Verification items for this drawing (mm, ordinates from the low corner). A direction names the side the tool comes from. Give positions to 0.01 mm unless a question says otherwise; leave off trailing zeros. Loops run counter-clockwise (first coordinate to the right, second up) from the corner with the lowest first, then second, coordinate; pieces in that order, holes last. Notation, with made-up numbers: (-33, -22.75) -> (10, -22.75) arc R18 cw to (10, 10.25) -> close; hole circle Ø7 at (26.25, -30). An arc over 180 degrees is marked (long way). Answer as a JSON object with one key per item and string values.
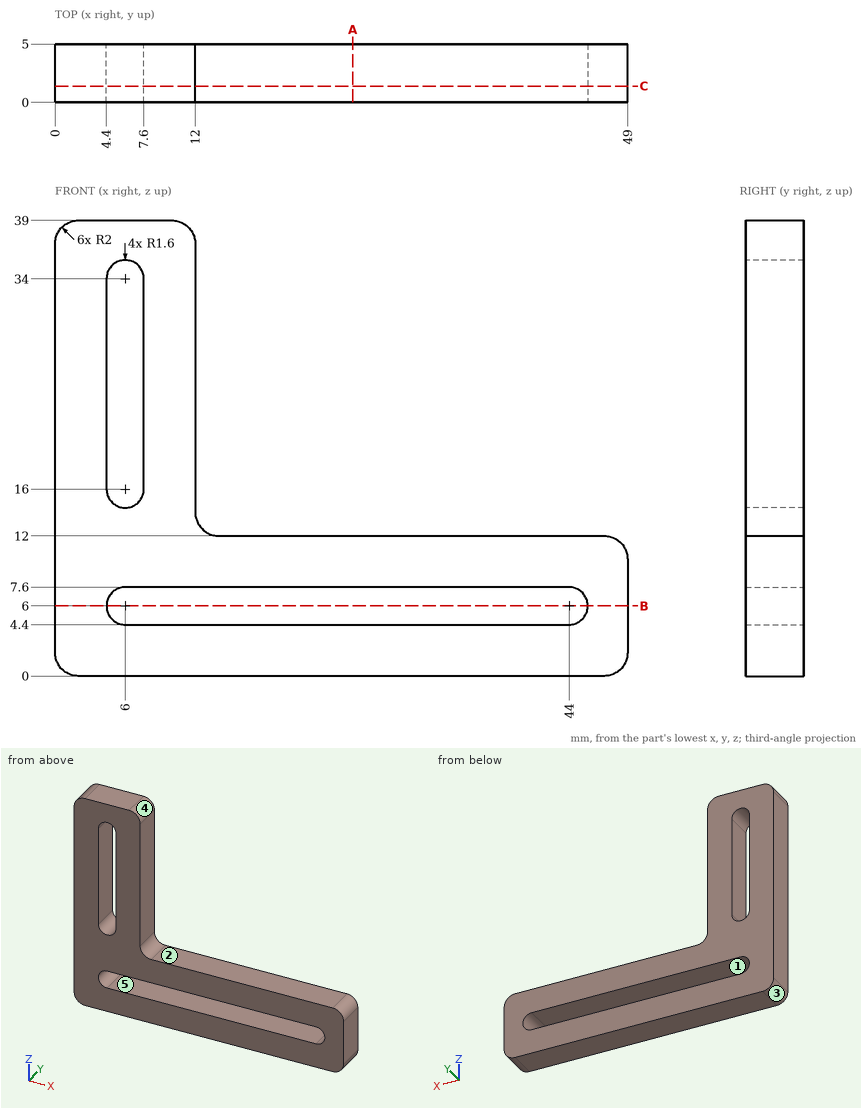
1) Tool access check on the marked faces 4 and 5. Record the directions out of +Z, -Z, +X, -X, +Y, -Y that give a thin tool (end or side, any length) a straight path to the whole face; none if there is none.
Geometry check:
{"face 4": "+Z, +X, +Y, -Y", "face 5": "+Y, -Y"}
2) Draft check along X on the marked faces 1, 2 and 3. Enter one of: pulls with the +X half, pulls with the -X half, needs draft (parallel to the pull), parting line crosses it, or undercut.
Geometry check:
{"face 1": "undercut", "face 2": "needs draft", "face 3": "pulls with the -X half"}
3) Section check A-A on x = 25.5. Record the cut outline in (y, z), plus the area to 3 significant figures.
Geometry check:
{"outline": "(0, 0) -> (5, 0) -> (5, 4.4) -> (0, 4.4) -> close; (0, 7.6) -> (5, 7.6) -> (5, 12) -> (0, 12) -> close", "area": "44.0 mm2"}
4) Material ranges on line 1 along X through (y, z) = (3.4, 24.5); line 2 along Z through (x, y) = (9, 2.5), recorded low to high. Write a range as from..to.
Geometry check:
{"line 1": "x = 0..4.4, 7.6..12", "line 2": "z = 0..4.4, 7.6..39"}
5) Section check B-B on z = 6. Record the cut outline in (x, y).
Geometry check:
{"outline": "(0, 0) -> (4.4, 0) -> (4.4, 5) -> (0, 5) -> close; (45.6, 0) -> (49, 0) -> (49, 5) -> (45.6, 5) -> close"}
6) Depth check by flat-ended pin: P1, Ø1.5, axis at x = 25, y = 2.5, coming from the +Z side; P2, Ø1.5, axis at y = 3, z = 22.5, coming from the +X side. Enter the tip coordinate at first touch or a pass-through.
Geometry check:
{"P1": "stops at z = 12", "P2": "stops at x = 12"}
7) Section check C-C on y = 1.4. Record the cut outline in (x, z), plus the area to 3 significant figures.
Geometry check:
{"outline": "(0, 2) arc R2 ccw to (2, 0) -> (47, 0) arc R2 ccw to (49, 2) -> (49, 10) arc R2 ccw to (47, 12) -> (14, 12) arc R2 cw to (12, 14) -> (12, 37) arc R2 ccw to (10, 39) -> (2, 39) arc R2 ccw to (0, 37) -> close; hole (4.4, 16) arc R1.6 ccw to (7.6, 16) -> (7.6, 34) arc R1.6 ccw to (4.4, 34) -> close; hole (6, 4.4) -> (44, 4.4) arc R1.6 ccw to (44, 7.6) -> (6, 7.6) arc R1.6 ccw to start", "area": "713 mm2"}
